CAD build for the part. Positions are in the model's coordinates, mm. Face numbers are marked on the shaded views. A direction names the side the tool comes from. Coordinates: 2 decimals unless noted, no trailing zeros. Write each loop counter-clockwise with the first axis right and the second up, starting at its lowest first coordinate (ties: lowest second). Pieces come first, ordered by that corner, then holes. Notation, with made-up numbers: (75.25, 57) - (128.25, 57) arc R22 ccw to (128.25, 74) - close; hole circle Ø9 at (-37, 52). An arc over 180 degrees is marked (long way). Answer in a Markdown table with one row per item. Add a question column.
Q1. Band-saw the part on B-B (x = -15). List the corners of the cut face in (y, z).
Q2. Drill centre lines: line 1 along Y through (x, z) = (-15, 16.75); line 2 along Y through (x, z) = (-15, 8); line 3 along Y through (x, z) = (-24, 38.5). Where is each one in solid material? Low to high. Write a range as from..to.
Q3. Band-saw the part on D-D (x = -54). List the corners of the cut face in (y, z), and give its area (3 significant figures).
Q4. Pin check, flat tips, straight feed: pin 1 (7 mm diameter, centred on x = -15, y = 88, fed in from -Z); pin 2 (5 mm diameter, centred on x = -21, z = 33.5, fed in from -Y); pin 3 (6 mm diameter, centred on x = -46.5, y = -90.5, fed in from +Z); pin 4 (13 mm diameter, centred on x = -15, y = -88, fed in from +Z). Stop position of each tip, or through.
Q5. Band-saw the part on C-C (z = 17.5). List the corners of the cut face in (x, y).
Q6. Band-saw the part on A-A (y = 88). List the corners of the cut face in (x, z), and give its area (3 significant figures).
Q7. 3-axis set-ups, long thin cutter, end or side, ignore diameter. For the marked faces 1, 2 and 3: which of +Z, -Z, +X, -X, +Y, -Y reach the whole face in a straight line?
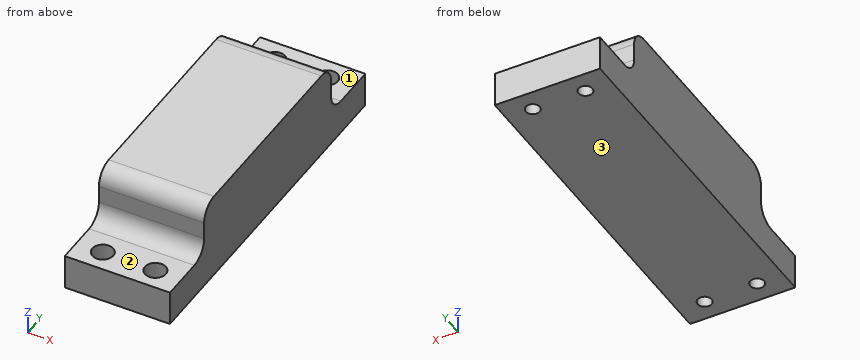
```python
from build123d import *

# Parameters (mm, degrees)
BOSS_EXTRUDE1_DEPTH                      = 60
CBORE_FOR_M10_HEX_HEAD_BOLT1_D           = 8
CBORE_FOR_M10_HEX_HEAD_BOLT1_CBORE_D     = 12
CBORE_FOR_M10_HEX_HEAD_BOLT1_CBORE_DEPTH = 10


with BuildPart() as part:
    # Sketch1 → Boss-Extrude1 (new body)
    with BuildSketch(Plane.YZ):
        with BuildLine():
            Line((-100, 0), (100, 0))
            Line((100, 0), (100, 20))
            Line((100, 20), (75, 20))
            ThreePointArc((75, 20), (67.928932188, 22.928932188), (65, 30))
            Line((65, 30), (65, 40))
            ThreePointArc((65, 40), (62.071067812, 47.071067812), (55, 50))
            Line((55, 50), (-55, 50))
            ThreePointArc((-55, 50), (-62.071067812, 47.071067812), (-65, 40))
            Line((-65, 40), (-65, 30))
            ThreePointArc((-65, 30), (-67.928932188, 22.928932188), (-75, 20))
            Line((-75, 20), (-100, 20))
            Line((-100, 20), (-100, 0))
        make_face()
    extrude(amount=-BOSS_EXTRUDE1_DEPTH)

    # CBORE for M10 Hex Head Bolt1 (through all)
    with Locations(Plane.XY.offset(20)):
        with Locations((-15, -88), (-45, -88), (-45, 88), (-15, 88)):
            CounterBoreHole(CBORE_FOR_M10_HEX_HEAD_BOLT1_D / 2, CBORE_FOR_M10_HEX_HEAD_BOLT1_CBORE_D / 2, CBORE_FOR_M10_HEX_HEAD_BOLT1_CBORE_DEPTH)


solid = part.part
```
Checked values:
| question | item | result |
|---|---|---|
| 1 | outline | (-100, 0) - (-92, 0) - (-92, 10) - (-94, 10) - (-94, 20) - (-100, 20) - close; (-84, 0) - (84, 0) - (84, 10) - (82, 10) - (82, 20) - (75, 20) arc R10 cw to (65, 30) - (65, 40) arc R10 ccw to (55, 50) - (-55, 50) arc R10 ccw to (-65, 40) - (-65, 30) arc R10 cw to (-75, 20) - (-82, 20) - (-82, 10) - (-84, 10) - close; (92, 0) - (100, 0) - (100, 20) - (94, 20) - (94, 10) - (92, 10) - close |
| 2 | line 1 | y = -100..-94, -82..82, 94..100 |
| 2 | line 2 | y = -100..-92, -84..84, 92..100 |
| 2 | line 3 | y = -65..65 |
| 3 | outline | (-100, 0) - (100, 0) - (100, 20) - (75, 20) arc R10 cw to (65, 30) - (65, 40) arc R10 ccw to (55, 50) - (-55, 50) arc R10 ccw to (-65, 40) - (-65, 30) arc R10 cw to (-75, 20) - (-100, 20) - close |
| 3 | area | 7,900 mm² |
| 4 | pin 1 | passes through |
| 4 | pin 2 | stops at y = -65 |
| 4 | pin 3 | stops at z = 10 |
| 4 | pin 4 | stops at z = 20 |
| 5 | outline | (-60, -100) - (0, -100) - (0, 100) - (-60, 100) - close; hole circle Ø12 at (-45, -88); hole circle Ø12 at (-45, 88); hole circle Ø12 at (-15, -88); hole circle Ø12 at (-15, 88) |
| 6 | outline | (-60, 0) - (-49, 0) - (-49, 10) - (-51, 10) - (-51, 20) - (-60, 20) - close; (-41, 0) - (-19, 0) - (-19, 10) - (-21, 10) - (-21, 20) - (-39, 20) - (-39, 10) - (-41, 10) - close; (-11, 0) - (0, 0) - (0, 20) - (-9, 20) - (-9, 10) - (-11, 10) - close |
| 6 | area | 800 mm² |
| 7 | face 1 | +Z, +X, -X, +Y |
| 7 | face 2 | +Z, +X, -X, -Y |
| 7 | face 3 | -Z, +X, -X, +Y, -Y |
